from build123d import *

# Parameters (mm, degrees)
SKETCH1_R           = 17
BOSS_EXTRUDE1_DEPTH = 25
SKETCH2_R           = 19
BOSS_EXTRUDE2_DEPTH = 8
BOSS_EXTRUDE3_DEPTH = 12
SKETCH4_R           = 16
BOSS_EXTRUDE4_DEPTH = 15


with BuildPart() as part:
    # Sketch1 → Boss-Extrude1 (new body)
    with BuildSketch(Plane.XY):
        Circle(SKETCH1_R)
    extrude(amount=BOSS_EXTRUDE1_DEPTH)

    # Sketch2 → Boss-Extrude2 (add)
    with BuildSketch(Plane(origin=(0, 0, 0), x_dir=(-1, 0, 0), z_dir=(0, 0, -1))):
        Circle(SKETCH2_R)
    extrude(amount=BOSS_EXTRUDE2_DEPTH)

    # Sketch3 → Boss-Extrude3 (add)
    with BuildSketch(Plane(origin=(0, 0, -8), x_dir=(-1, 0, 0), z_dir=(0, 0, -1))):
        with BuildLine():
            ThreePointArc((-43.790428919, -14.085394388), (-33.713723077, 16.075398615), (-13.776954685, 40.84914886))
            ThreePointArc((-13.776954685, 40.84914886), (-0.147298901, 45.999483399), (13.55326526, 41.040854117))
            ThreePointArc((13.55326526, 41.040854117), (33.645906333, 16.883464851), (44.209571081, -12.708808948))
            ThreePointArc((44.209571081, -12.708808948), (0.719490727, -45.994372842), (-43.790428919, -14.085394388))
        make_face()
    extrude(amount=BOSS_EXTRUDE3_DEPTH)

    # Sketch4 → Boss-Extrude4 (add)
    with BuildSketch(Plane(origin=(0, 0, -20), x_dir=(-1, 0, 0), z_dir=(0, 0, -1))):
        with Locations((0, 25)):
            Circle(SKETCH4_R)
    extrude(amount=BOSS_EXTRUDE4_DEPTH)

    # Mirror1: part across plane


with BuildPart() as part_1:
    add(part.part)
    add(part.part.mirror(Plane(origin=(0, 25, -35), x_dir=(1, 0, 0), z_dir=(0, 0, -1))))


solid = part_1.part
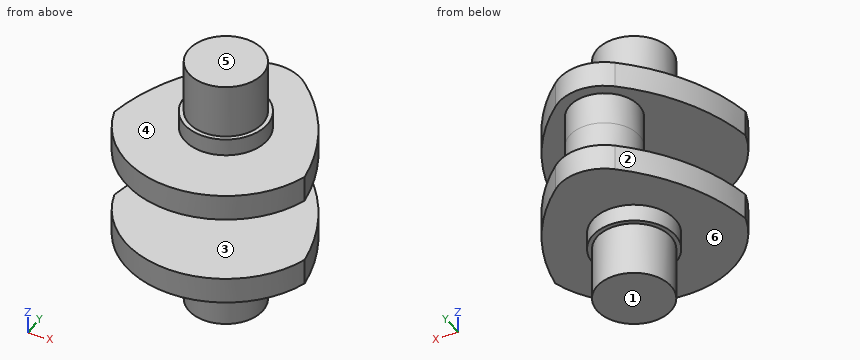
Source: CAD feature listing. Evaluate the final solid. Frame: model axes, mm. Face numbers are marked on the shaded views. A direction names the side the tool comes from. Give positions to 0.01 mm unless a question says otherwise; leave off trailing zeros. Write each loop counter-clockwise with the first axis right and the second up, starting at its lowest first coordinate (ties: lowest second). Pieces come first, ordered by that corner, then holes. Notation, with made-up numbers: M -23,19.25 L 20,19.25 A27 ccw 20,37.25 Z; hole C 47,22.5 d3. An arc over 180 degrees is marked long. Return JSON: item names as keys, results as strings. Group by question number.
1) Material intervals for line 1 along Z through (x, y) = (-2.5, 41.5); line 2 along Z through (x, y) = (-17.5, -3.5); line 3 along Z through (x, y) = (0, 26.5), sorted ascending. Write a range as [from, to].
2) Pin query (flat end, axial travel): P1, Ø1, axis at x = 2.5, z = -16, coming from the -Y side; P2, Ø1.5, axis at y = -24, z = -52.5, coming from the +X side; P3, Ø10, axis at y = -21.5, z = -59, coming from the -X side. Return the tip coordinate at first contact, or that it passes through.
3) Cut plane A-A, the plane y = -21. Output: boundary loops of the cut face in (x, z), plus the area to 3 significant figures.
4) Pull-direction query (Z, two-part tool) for the marked faces 1, 2 and 3; classes: pulls with the +Z half, pulls with the -Z half, needs draft (parallel to the pull), parting line crosses it, or undercut.
5) Set-up query: the marked faces 4, 5 and 6. Return all of +Z, -Z, +X, -X, +Y, -Y with unobstructed straight access to the full face (end or side cutting, diameter ignored); none if empty.
6) Cut plane B-B, the plane x = 0. Output: boundary loops of the cut face in (y, z).
7) Cut plane D-D, the plane z = -58. Output: boundary loops of the cut face in (x, y).
8) Cut plane C-C, the plane x = -35. Output: boundary loops of the cut face in (y, z), plus the area to 3 significant figures.
Recorded:
{
 "1": {"line 1": "z = [-62, -50], [-20, -8]", "line 2": "z = [-70, -50], [-20, 0]", "line 3": "z = [-62, -8]"},
 "2": {"P1": "stops at y = -45.96", "P2": "stops at x = 39.69", "P3": "stops at x = -42.94"},
 "3": {"outline": "M -40.93,-62 L 40.93,-62 L 40.93,-50 L -40.93,-50 Z; M -40.93,-20 L 40.93,-20 L 40.93,-8 L -40.93,-8 Z", "area": "1,960 mm²"},
 "4": {"face 1": "pulls with the -Z half", "face 2": "needs draft", "face 3": "undercut"},
 "5": {"face 4": "+Z", "face 5": "+Z, +X, -X, +Y, -Y", "face 6": "-Z"},
 "6": {"outline": "M -46,-62 L -19,-62 L -19,-70 L -17,-70 L -17,-95 L 17,-95 L 17,-70 L 19,-70 L 19,-62 L 46,-62 L 46,-50 L 41,-50 L 41,-20 L 46,-20 L 46,-8 L 19,-8 L 19,0 L 17,0 L 17,25 L -17,25 L -17,0 L -19,0 L -19,-8 L -46,-8 L -46,-20 L 9,-20 L 9,-50 L -46,-50 Z"},
 "7": {"outline": "M -44.21,-12.71 A46 ccw 43.79,-14.09 A90 ccw 13.78,40.85 A21 ccw -13.55,41.04 A90 ccw Z"},
 "8": {"outline": "M -29.85,-62 L 14.42,-62 L 14.42,-50 L -29.85,-50 Z; M -29.85,-20 L 14.42,-20 L 14.42,-8 L -29.85,-8 Z", "area": "1,060 mm²"}
}
